from build123d import *

# Parameters (mm, degrees)
SKETCH1_R          = 4.7625
EXTRUDE1_DEPTH     = 25.4
SKETCH3_R          = 7.9375
EXTRUDE3_DEPTH     = 4.7625
CHAMFER1_SIZE      = 0.762
CUT_EXTRUDE1_DEPTH = 4.064


with BuildPart() as part:
    # Sketch1 → Extrude1 (new body)
    with BuildSketch(Plane.XY):
        Circle(SKETCH1_R)
    extrude(amount=EXTRUDE1_DEPTH)

    # Sketch3 → Extrude3 (add)
    with BuildSketch(Plane.XY.offset(25.4)):
        with Locations((0, 0.491553118)):
            Circle(SKETCH3_R)
    extrude(amount=EXTRUDE3_DEPTH)

    # Chamfer1
    chamfer1_edges = [part.edges().sort_by_distance(p)[0] for p in [
        (-7.9375, 0.491553118, 30.1625),
        (-4.7625, 0, 0),
    ]]
    chamfer(chamfer1_edges, length=CHAMFER1_SIZE)

    # Sketch4 → Cut-Extrude1 (cut)
    with BuildSketch(Plane.XY.offset(30.1625)):
        Polygon((5.08, 0), (2.54, 4.399409051), (-2.54, 4.399409051), (-5.08, 0), (-2.54, -4.399409051), (2.54, -4.399409051), align=None)
    extrude(amount=-CUT_EXTRUDE1_DEPTH, mode=Mode.SUBTRACT)


solid = part.part
Source: CAD feature listing. Evaluate the final solid. Frame: model axes, mm. A direction names the side the tool comes from. Give positions to 0.01 mm unless a question says otherwise; leave off trailing zeros. Write each loop counter-clockwise with the first axis right and the second up, starting at its lowest first coordinate (ties: lowest second). Pieces come first, ordered by that corner, then holes. Notation, with made-up numbers: M -39,-32.5 L -26,-32.5 A12 ccw -26,-13.5 Z; hole C 54.5,49.5 d4. An arc over 180 degrees is marked long. Return JSON: item names as keys, results as strings. Group by question number.
1) First-contact query: pin 1 Ø6 at (x, z) = (-5, 17) entering from -Y; pin 2 Ø4 at (y, z) = (6.5, 26.5) entering from +X; pin 3 Ø4 at (y, z) = (-2.5, 12.5) entering from +X. Flat tips, straight axial feed; report the tip coordinate or a pass-through.
2) Cut plane B-B, the plane z = 4. Output: boundary loops of the cut face in (x, y) (1 decimal).
3) Ray query, L1, parallel to Z at x = 6, y = 3.5; L2, parallel to X at y = -0.5, z = 27; L3, parallel to Z at x = 2, y = 3. Return the intervals inside material, ascending.
4) Draft query along Y for faces 1 (the face through (3, 4, 25.4)), 2 (the face through (0, 4.399, 28)), 3 (the face through (7.57, 2.88, 27.37)). Return one class per face: released by +Y, released by -Y, zero draft, split by the parting line, or undercut.
5) Set-up query: faces 4 (the face through (-3.828, -2.169, 28.159)), 5 (the face through (-3.78, -2.9, 12.91)), 6 (the face through (0, 0, 0)). Return all of +Z, -Z, +X, -X, +Y, -Y with unobstructed straight access to the full face (end or side cutting, diameter ignored); none if empty.
6) Cut plane A-A, the plane x = 0. Output: boundary loops of the cut face in (y, z).
Data:
{
 "1": {"pin 1": "stops at y = -4.32", "pin 2": "stops at x = 6.85", "pin 3": "stops at x = 4.74"},
 "2": {"outline": "C 0,0 d9.5"},
 "3": {"L1": "z = 25.4 to 30.16", "L2": "x = -7.88 to -4.79, 4.79 to 7.88", "L3": "z = 0 to 26.1"},
 "4": {"face 1": "zero draft", "face 2": "undercut", "face 3": "split by the parting line"},
 "5": {"face 4": "+Z", "face 5": "-Z", "face 6": "-Z, +X, -X, +Y, -Y"},
 "6": {"outline": "M -7.45,25.4 L -4.76,25.4 L -4.76,0.76 L -4,0 L 4,0 L 4.76,0.76 L 4.76,25.4 L 8.43,25.4 L 8.43,29.4 L 7.67,30.16 L 4.4,30.16 L 4.4,26.1 L -4.4,26.1 L -4.4,30.16 L -6.68,30.16 L -7.45,29.4 Z"}
}
